from build123d import *

# Parameters (mm, degrees)
F0_R     = 6.4
F1_DEPTH = 22.15
F2_R     = 5.5
F2_R_2   = 3
F3_DEPTH = 9


with BuildPart() as f1:
    # F0 (on Front) → F1 (new body)
    with BuildSketch(Plane.XZ):
        Circle(F0_R)
    extrude(amount=F1_DEPTH)

    # F2 (on face) → F3 (join)
    with BuildSketch(Plane(origin=(0, 0, 0), x_dir=(-1, 0, 0), z_dir=(0, 1, 0))):
        Circle(F2_R)
        Circle(F2_R_2, mode=Mode.SUBTRACT)
    extrude(amount=F3_DEPTH)


solid = f1.part
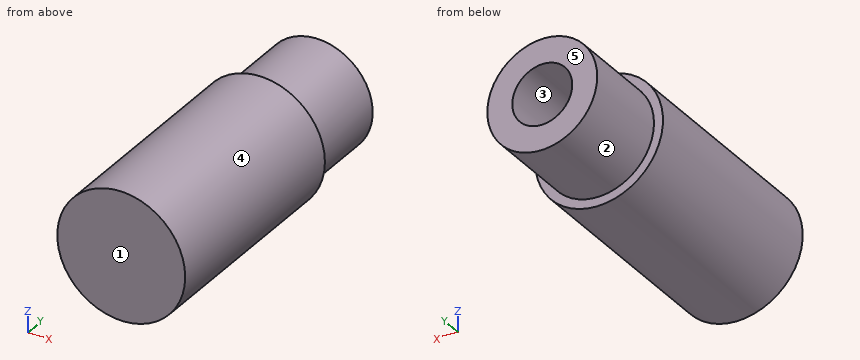
Design review of the part built by this model. Coordinates are the model's own, in mm. Face numbers are marked on the shaded views. A direction names the side the tool comes from. Give positions to 0.01 mm unless a question says otherwise; leave off trailing zeros. Order: outer loops, then holes, each group sorted by start corner. A loop starts at its lowest first (then second) coordinate and runs counter-clockwise, first axis right, second up. Notation, with made-up numbers: (-38, -35) - (20, -35) arc R21 cw to (20, -15) - close; hole circle Ø3 at (-17.5, -17). An arc over 180 degrees is marked (long way). Write item = value, one per line. Start each with the question number.
Q1. Clearance check with flat-ended pins moving along their axes: pin 1 Ø1 at (x, y) = (-0.5, 1) entering from +Z; pin 2 Ø5 at (y, z) = (-6.5, 5) entering from +X; pin 3 Ø1.5 at (x, y) = (-2, -5) entering from +Z. State where each tip first meets the part, or that it passes through.
Q2. We need section C-C on y = -8. State the section outline as (x, z) points.
Q3. Mouldability with a two-part tool opening along X and no side actions: class the marked faces 3, 4 and 5 as released by +X, released by -X, zero draft, split by the parting line, or undercut.
Q4. We need section A-A on z = 0. State the section outline as (x, y) points, plus the area to 3 significant figures.
Q5. Tool access review of the marked faces 1 and 2: name each direction out of +Z, -Z, +X, -X, +Y, -Y from which nothing blocks a thin tool from reaching the whole face with its end or side.
Q6. We need section D-D on z = 4.5. State the section outline as (x, y) points, plus the area to 3 significant figures.
Q7. We need section B-B on x = 0. State the section outline as (y, z) points.
Q8. To check wall thickness, follow L1, parallel to Z at x = 0, y = 7.25; L2, parallel to Y at x = 4.5, z = -3.75; L3, parallel to X at y = 5, z = 1.5. State the ranges of each line that lie inside material, in increasing order. Write a range as from..to.
Working result:
q1.pin_1 = 5.5
q1.pin_2 = 5.89
q1.pin_3 = 6.28
q2.outline = circle Ø12.8 at (0, 0)
q3.face_3 = undercut
q3.face_4 = split by the parting line
q3.face_5 = zero draft
q4.outline = (-6.4, -22.15) - (6.4, -22.15) - (6.4, 0) - (5.5, 0) - (5.5, 9) - (3, 9) - (3, 0) - (-3, 0) - (-3, 9) - (-5.5, 9) - (-5.5, 0) - (-6.4, 0) - close
q4.area = 329 mm²
q5.face_1 = +Z, -Z, +X, -X, -Y
q5.face_2 = +Y
q6.outline = (-4.55, -22.15) - (4.55, -22.15) - (4.55, 0) - (3.16, 0) - (3.16, 9) - (-3.16, 9) - (-3.16, 0) - (-4.55, 0) - close
q6.area = 259 mm²
q7.outline = (-22.15, -6.4) - (0, -6.4) - (0, -5.5) - (9, -5.5) - (9, -3) - (0, -3) - (0, 3) - (9, 3) - (9, 5.5) - (0, 5.5) - (0, 6.4) - (-22.15, 6.4) - close
q8.L1 = -5.5..-3, 3..5.5
q8.L2 = -22.15..0
q8.L3 = -5.29..-2.6, 2.6..5.29
